```python
from build123d import *

# Parameters (mm, degrees)
F1_DEPTH = 23.0124
F2_R     = 2.778125
F3_DEPTH = 23.0124
F4_W     = 11.5062
F4_H     = 19.2024
F5_DEPTH = 39.3931387462
F6_W     = 11.0744
F6_H     = 19.2024
F7_DEPTH = 15.3162
F8_SIZE  = 1.90499


# Not quite as in the source:
# - a fillet or chamfer is up to 0.001 mm smaller than in the source, because OpenCascade refuses the exact size


with BuildPart() as f1:
    # F0 (on Top) → F1 (new body)
    with BuildSketch(Plane.XY):
        with BuildLine():
            Line((-13.9381455007, -23.59), (13.9381455007, -23.59))
            ThreePointArc((13.9381455007, -23.59), (19.3747258045, -19.3747258045), (23.59, -13.9381455007))
            Line((23.59, -13.9381455007), (23.59, 13.9381455007))
            ThreePointArc((23.59, 13.9381455007), (19.3747258045, 19.3747258045), (13.9381455007, 23.59))
            Line((13.9381455007, 23.59), (-13.9381455007, 23.59))
            ThreePointArc((-13.9381455007, 23.59), (-19.3747258045, 19.3747258045), (-23.59, 13.9381455007))
            Line((-23.59, 13.9381455007), (-23.59, -13.9381455007))
            ThreePointArc((-23.59, -13.9381455007), (-19.3747258045, -19.3747258045), (-13.9381455007, -23.59))
        make_face()
        with BuildLine():
            ThreePointArc((13.3802802661, 21.59), (17.9605122421, 17.9605122421), (21.59, 13.3802802661))
            Line((21.59, 13.3802802661), (21.59, -13.3802802661))
            ThreePointArc((21.59, -13.3802802661), (17.9605122421, -17.9605122421), (13.3802802661, -21.59))
            Line((13.3802802661, -21.59), (-13.3802802661, -21.59))
            ThreePointArc((-13.3802802661, -21.59), (-17.9605122421, -17.9605122421), (-21.59, -13.3802802661))
            Line((-21.59, -13.3802802661), (-21.59, 13.3802802661))
            ThreePointArc((-21.59, 13.3802802661), (-17.9605122421, 17.9605122421), (-13.3802802661, 21.59))
            Line((-13.3802802661, 21.59), (13.3802802661, 21.59))
        make_face(mode=Mode.SUBTRACT)
    extrude(amount=F1_DEPTH)

    # F2 (on Top) → F3 (join, through all)
    with BuildSketch(Plane.XY):
        with BuildLine():
            Line((15.5641722456, 37.4711913278), (9.0912664251, 23.59))
            Line((9.0912664251, 23.59), (19.6607342764, 18.6613761983))
            ThreePointArc((19.6607342764, 18.6613761983), (29.8377828505, 22.365518952), (26.1336400968, 32.5425675261))
            Line((26.1336400968, 32.5425675261), (15.5641722456, 37.4711913278))
        make_face()
        with Locations((22.7869465963, 25.3655601533)):
            Circle(F2_R, mode=Mode.SUBTRACT)
    extrude(amount=F3_DEPTH)

    # F4 (on face) → F5 (cut, through all)
    with BuildSketch(Plane(origin=(-1.5679842868, 0.7311630808, 0), x_dir=(-0.4226182617, -0.906307787, 0), z_dir=(-0.906307787, 0.4226182617, 0))):
        with Locations((-32.8800359098, 11.5062)):
            Rectangle(F4_W, F4_H)
    extrude(amount=-F5_DEPTH, mode=Mode.SUBTRACT)

    # F6 (on face) → F7 (cut)
    with BuildSketch(Plane(origin=(17.1321565324, 36.740028247, 0), x_dir=(-0.906307787, 0.4226182617, 0), z_dir=(0.4226182617, 0.906307787, 0))):
        with Locations((-12.0529382029, 11.5062)):
            Rectangle(F6_W, F6_H)
    extrude(amount=-F7_DEPTH, mode=Mode.SUBTRACT)

    # F8 (size 1.905 in the source; OpenCascade refuses exactly that, so slightly less here)
    f8_edges = [f1.edges().sort_by_distance(p)[0] for p in [
        (17.369603, 21.831683, 11.5062),
        (22.232333, 32.259842, 11.5062),
    ]]
    chamfer(f8_edges, length=F8_SIZE)


solid = f1.part
```
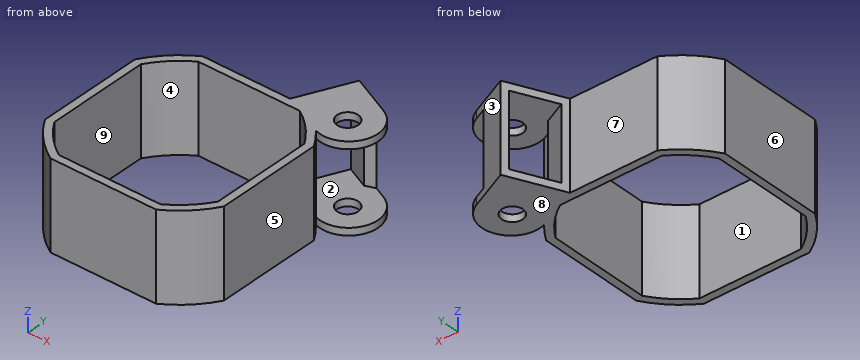
The model under review builds one solid part; all positions refer to its coordinate system, in mm. Face numbers are marked on the shaded views. A direction names the side the tool comes from. Give positions to 0.01 mm unless a question says otherwise; leave off trailing zeros. Write each loop counter-clockwise with the first axis right and the second up, starting at its lowest first coordinate (ties: lowest second). Pieces come first, ordered by that corner, then holes. Notation, with made-up numbers: (-5, -14) -> (33, -14) arc R32 ccw to (33, 21) -> close; hole circle Ø8 at (16, -31). An arc over 180 degrees is marked (long way). Put each result on its own line as item: value.
(1) We need section B-B, the plane x = 1. Give the boundary of the cut face in (y, z).
Results are:
outline: (-23.59, 0) -> (-21.59, 0) -> (-21.59, 23.01) -> (-23.59, 23.01) -> close; (21.59, 0) -> (23.59, 0) -> (23.59, 23.01) -> (21.59, 23.01) -> close
(2) For pin 1 Ø11.5 at (x, z) = (1.5, 13.5) entering from +Y; pin 2 Ø5 at (x, y) = (22.79, 25.37) entering from +Z; pin 3 Ø5 at (y, z) = (-9.5, 12.5) entering from +X; pin 4 Ø4 at (y, z) = (26, 8) entering from -X, all flat-tipped, find the tip position at first contact; note any pin that passes through.
Results are:
pin 1: y = 23.59
pin 2: through
pin 3: x = 23.59
pin 4: x = 9.28
(3) The part is to be moulded in two halves that separate along X. For the marked faces 1, 2, 3 and 4, say which applies: pulls with the +X half, pulls with the -X half, needs draft (parallel to the pull), parting line crosses it, or undercut.
Results are:
face 1: undercut
face 2: needs draft
face 3: pulls with the +X half
face 4: undercut
(4) Tool access review of the marked faces 5, 6, 7, 8 and 9: name each direction out of +Z, -Z, +X, -X, +Y, -Y from which nothing blocks a thin tool from reaching the whole face with its end or side.
Results are:
face 5: +Z, -Z, +X, -Y
face 6: +Z, -Z, -X, +Y, -Y
face 7: +Z, -Z, -X, +Y
face 8: -Z, +X, -X, +Y, -Y
face 9: +Z, -Z
(5) We need section D-D, the plane x = 24.5. Give the boundary of the cut face in (y, z) (3 decimals).
Results are:
outline: (18.113, 0) -> (23.178, 0) -> (23.178, 1.905) -> (18.113, 1.905) -> close; (18.113, 21.107) -> (23.178, 21.107) -> (23.178, 23.012) -> (18.113, 23.012) -> close; (27.553, 0) -> (33.304, 0) -> (33.304, 1.905) -> (27.553, 1.905) -> close; (27.553, 21.107) -> (33.304, 21.107) -> (33.304, 23.012) -> (27.553, 23.012) -> close
(6) We need section A-A, the plane z = 13.75. State how many separate pieces and enclosed holes the cut face has, and give its area (3 significant figures).
Results are:
separate pieces: 2
enclosed holes: 1
area: 334 mm²
(7) To check wall thickness, follow probe 1 along Y at (x, z) = (4.5, 4); probe 2 along Z at (x, y) = (27.5, 28.5) (3 decimals). State the ranges of each line that lie inside material, in increasing order. Write a range as from..to.
Results are:
probe 1: -23.59..-21.59, 21.59..23.59
probe 2: 0..1.905, 21.107..23.012
